Work out the finished part from the listing and answer in its coordinate system (mm). A direction names the side the tool comes from. Round coordinates to 2 decimals unless told otherwise and drop trailing zeros. Loops run counter-clockwise (first coordinate to the right, second up) from the corner with the lowest first, then second, coordinate; pieces in that order, holes last.
from build123d import *

# Parameters (mm, degrees)
F0_W     = 25
F0_H     = 77
F1_DEPTH = 5
F2_R     = 1.5
F3_DEPTH = 50
F4_R     = 5
F5_W     = 4
F5_H     = 77
F6_DEPTH = 4


with BuildPart() as f1:
    # F0 (on Top) → F1 (new body)
    with BuildSketch(Plane.XY):
        with BuildLine():
            ThreePointArc((0, 5), (1.4644660941, 1.4644660941), (5, 0))
            Line((5, 0), (135, 0))
            ThreePointArc((135, 0), (138.5355339059, 1.4644660941), (140, 5))
            Line((140, 5), (140, 90))
            ThreePointArc((140, 90), (138.5355339059, 93.5355339059), (135, 95))
            Line((135, 95), (5, 95))
            ThreePointArc((5, 95), (1.4644660941, 93.5355339059), (0, 90))
            Line((0, 90), (0, 5))
        make_face()
        with Locations((41.5, 47.5)):
            Rectangle(F0_W, F0_H, mode=Mode.SUBTRACT)
    extrude(amount=F1_DEPTH)

    # F2 (on face) → F3 (join)
    with BuildSketch(Plane.XY.offset(5)):
        with BuildLine():
            ThreePointArc((0, 5), (1.4644660941, 1.4644660941), (5, 0))
            Line((5, 0), (135, 0))
            ThreePointArc((135, 0), (138.5355339059, 1.4644660941), (140, 5))
            Line((140, 5), (140, 90))
            ThreePointArc((140, 90), (138.5355339059, 93.5355339059), (135, 95))
            Line((135, 95), (5, 95))
            ThreePointArc((5, 95), (1.4644660941, 93.5355339059), (0, 90))
            Line((0, 90), (0, 5))
        make_face()
        with Locations((5, 5)):
            Circle(F2_R, mode=Mode.SUBTRACT)
        with Locations((135, 5)):
            Circle(F2_R, mode=Mode.SUBTRACT)
        with Locations((5, 90)):
            Circle(F2_R, mode=Mode.SUBTRACT)
        Polygon((10, 9.9999997765), (5, 9.9999997765), (5, 85), (10, 85), (10, 90), (130, 90), (130, 85), (135, 85), (135, 9.9999997765), (130, 9.9999997765), (130, 5), (10, 5), align=None, mode=Mode.SUBTRACT)
        with Locations((135, 90)):
            Circle(F2_R, mode=Mode.SUBTRACT)
    extrude(amount=F3_DEPTH)

    # F4
    f4_edges = [f1.edges().sort_by_distance(p)[0] for p in [
        (70, 95, 0),
    ]]
    fillet(f4_edges, radius=F4_R)

    # F5 (on face) → F6 (join)
    with BuildSketch(Plane.XY.offset(5)):
        with Locations((27, 47.5)):
            Rectangle(F5_W, F5_H)
        with Locations((56, 47.5)):
            Rectangle(F5_W, F5_H)
    extrude(amount=F6_DEPTH)


solid = f1.part
Item 1: Section D-D, the plane x = 62 is taken. Give the vertices of the cut face in (y, z).
Item 2: Section A-A, the plane y = 66.5 is taken. Give the vertices of the cut face in (x, z).
Item 3: Straight lines are drawn through the part: line 1 (X direction, y = 16, z = 6); line 2 (Y direction, x = 99, z = 45); line 3 (X direction, y = 38, z = 33). For each, find the intervals that lie inside material, in ascending order.
Item 4: Determine the mould class of faces 1 (the face through (71, 95, 30)), 2 (the face through (56, 86, 7)), 3 (the face through (139, 93, 30)) for opening direction X: pulls with the +X half, pulls with the -X half, needs draft (parallel to the pull), parting line crosses it, or undercut.
Item 5: For faces 4 (the face through (138, 48, 1)), 5 (the face through (29, 47, 4)), 6 (the face through (133, 10, 30)), determine the directions among +Z, -Z, +X, -X, +Y, -Y from which every point of the face is accessible in a straight line to the end or side of a thin tool.
Item 6: Section C-C, the plane z = 41 is taken. Give the vertices of the cut face in (x, y), plus the area to 3 significant figures.
Item 7: Each of these flat-tipped pins is pushed along its axis until it touches: P1, Ø1.5, axis at x = 5, y = 89.5, coming from the +Z side; P2, Ø3, axis at x = 26, y = 61, coming from the +Z side. Where does it stop, or does it pass through?
Item 8: Section B-B, the plane x = 32 is taken. Give the vertices of the cut face in (y, z), plus the area to 3 significant figures.
Answer below:
1. outline: (0, 5) arc R5 ccw to (5, 0) - (90, 0) arc R5 ccw to (95, 5) - (95, 55) - (90, 55) - (90, 5) - (5, 5) - (5, 55) - (0, 55) - close
2. outline: (0, 5) arc R5 ccw to (5, 0) - (29, 0) - (29, 9) - (25, 9) - (25, 5) - (5, 5) - (5, 55) - (0, 55) - close; (54, 0) - (135, 0) arc R5 ccw to (140, 5) - (140, 55) - (135, 55) - (135, 5) - (58, 5) - (58, 9) - (54, 9) - close
3. line 1: x = 0 to 5, 25 to 29, 54 to 58, 135 to 140
3. line 2: y = 0 to 5, 90 to 95
3. line 3: x = 0 to 5, 135 to 140
4. face 1: needs draft
4. face 2: undercut
4. face 3: pulls with the +X half
5. face 4: -Z, +X, +Y, -Y
5. face 5: +Z, -Z
5. face 6: +Z
6. outline: (0, 5) arc R5 ccw to (5, 0) - (135, 0) arc R5 ccw to (140, 5) - (140, 90) arc R5 ccw to (135, 95) - (5, 95) arc R5 ccw to (0, 90) - close; hole circle Ø3 at (5, 5); hole circle Ø3 at (5, 90); hole (5, 10) - (10, 10) - (10, 5) - (130, 5) - (130, 10) - (135, 10) - (135, 85) - (130, 85) - (130, 90) - (10, 90) - (10, 85) - (5, 85) - close; hole circle Ø3 at (135, 5); hole circle Ø3 at (135, 90)
6. area: 2,300 mm2
7. P1: stops at z = 5
7. P2: stops at z = 9
8. outline: (0, 5) arc R5 ccw to (5, 0) - (9, 0) - (9, 5) - (5, 5) - (5, 55) - (0, 55) - close; (86, 0) - (90, 0) arc R5 ccw to (95, 5) - (95, 55) - (90, 55) - (90, 5) - (86, 5) - close
8. area: 579 mm2
